```python
from build123d import *

# Parameters (mm, degrees)
SKETCH1_W                    = 129
SKETCH1_H                    = 107.4
SKETCH1_R                    = 1.65
BOSS_EXTRUDE1_DEPTH          = 3
BOSS_EXTRUDE2_DEPTH          = 5
BOSS_EXTRUDE3_START          = 5
SKETCH2_R                    = 4
SKETCH2_R_2                  = 1.6
BOSS_EXTRUDE3_DEPTH          = 5
CUT_EXTRUDE1_START           = 3
CUT_EXTRUDE1_OUTLINE_R       = 1.6
CUT_EXTRUDE1_DEPTH           = 2
FILLET3_R                    = 2
FILLET4_R                    = 2
SKETCH1_4_R                  = 2.407849471
CUT_EXTRUDE2_DEPTH           = 1
CUT_EXTRUDE2_DRAFT           = 45
CUT_EXTRUDE2_PROFILE_2_DEPTH = 1
CUT_EXTRUDE2_PROFILE_2_DRAFT = 45
CUT_EXTRUDE2_PROFILE_3_DEPTH = 1
CUT_EXTRUDE2_PROFILE_3_DRAFT = 45
CUT_EXTRUDE2_PROFILE_4_DEPTH = 1
CUT_EXTRUDE2_PROFILE_4_DRAFT = 45
CHAMFER1_SIZE                = 1.5


# Read off the part's stored shape, not the designer's step: Cut-Extrude1
with BuildPart() as part:
    # Sketch1 → Boss-Extrude1 (new body)
    with BuildSketch(Plane(origin=(0, 0, 0), x_dir=(1, 0, 0), z_dir=(0, 1, 0))):
        Rectangle(SKETCH1_W, SKETCH1_H)
        with Locations(Location((-60.3, -49.5, 0), (0, 0, 270))):
            Circle(SKETCH1_R, mode=Mode.SUBTRACT)
        with Locations(Location((60.3, -49.5, 0), (0, 0, 270))):
            Circle(SKETCH1_R, mode=Mode.SUBTRACT)
        with Locations(Location((-60.3, 49.5, 0), (0, 0, 270))):
            Circle(SKETCH1_R, mode=Mode.SUBTRACT)
        Polygon((49.912004588, -49.253731343), (-49.912004588, -49.253731343), (-60, -39.165735931), (-60, 39.165735931), (-49.912004588, 49.253731343), (49.912004588, 49.253731343), (60, 39.165735931), (60, -39.165735931), align=None, mode=Mode.SUBTRACT)
        with Locations(Location((60.3, 49.5, 0), (0, 0, 270))):
            Circle(SKETCH1_R, mode=Mode.SUBTRACT)
    extrude(amount=BOSS_EXTRUDE1_DEPTH)

    # Sketch1<3> → Boss-Extrude2 (add)
    with BuildSketch(Plane(origin=(0, 0, 0), x_dir=(1, 0, 0), z_dir=(0, 1, 0))):
        Polygon((-49.912004588, 49.253731343), (-60, 39.165735931), (-60, -39.165735931), (-49.912004588, -49.253731343), (49.912004588, -49.253731343), (60, -39.165735931), (60, 39.165735931), (49.912004588, 49.253731343), align=None)
    extrude(amount=BOSS_EXTRUDE2_DEPTH)

    # Sketch2 → Boss-Extrude3 (add)
    # profile 1 of 4: a face of its own
    with BuildSketch(Plane(origin=(0, 0, 0), x_dir=(1, 0, 0), z_dir=(0, 1, 0)).offset(BOSS_EXTRUDE3_START)):
        with Locations(Location((-39.313021369, -41.297235267, 0), (0, 0, 270))):
            Circle(SKETCH2_R)
        with Locations(Location((-39.313021369, -41.297235267, 0), (0, 0, 270))):
            Circle(SKETCH2_R_2, mode=Mode.SUBTRACT)
    # profile 2 of 4: a face of its own
    with BuildSketch(Plane(origin=(0, 0, 0), x_dir=(1, 0, 0), z_dir=(0, 1, 0)).offset(BOSS_EXTRUDE3_START)):
        with Locations(Location((36.886978631, 6.962764733, 0), (0, 0, 270))):
            Circle(SKETCH2_R)
        with Locations(Location((36.886978631, 6.962764733, 0), (0, 0, 270))):
            Circle(SKETCH2_R_2, mode=Mode.SUBTRACT)
    # profile 3 of 4: a face of its own
    with BuildSketch(Plane(origin=(0, 0, 0), x_dir=(1, 0, 0), z_dir=(0, 1, 0)).offset(BOSS_EXTRUDE3_START)):
        with Locations(Location((-38.043021369, 6.962764733, 0), (0, 0, 270))):
            Circle(SKETCH2_R)
        with Locations(Location((-38.043021369, 6.962764733, 0), (0, 0, 270))):
            Circle(SKETCH2_R_2, mode=Mode.SUBTRACT)
    # profile 4 of 4: a face of its own
    with BuildSketch(Plane(origin=(0, 0, 0), x_dir=(1, 0, 0), z_dir=(0, 1, 0)).offset(BOSS_EXTRUDE3_START)):
        with Locations(Location((43.236978631, -41.297235267, 0), (0, 0, 270))):
            Circle(SKETCH2_R)
        with Locations(Location((43.236978631, -41.297235267, 0), (0, 0, 270))):
            Circle(SKETCH2_R_2, mode=Mode.SUBTRACT)
    extrude(amount=BOSS_EXTRUDE3_DEPTH)

    # Cut-Extrude1 outline → Cut-Extrude1 (cut)
    with BuildSketch(Plane(origin=(0, 0, 0), x_dir=(1, 0, 0), z_dir=(0, 1, 0)).offset(CUT_EXTRUDE1_START)):
        with Locations((-38.043021369, 6.962764733)):
            Circle(CUT_EXTRUDE1_OUTLINE_R)
        with Locations((-39.313021369, -41.297235267)):
            Circle(CUT_EXTRUDE1_OUTLINE_R)
        with Locations((43.236978631, -41.297235267)):
            Circle(CUT_EXTRUDE1_OUTLINE_R)
        with Locations((36.886978631, 6.962764733)):
            Circle(CUT_EXTRUDE1_OUTLINE_R)
    extrude(amount=CUT_EXTRUDE1_DEPTH, mode=Mode.SUBTRACT)

    # Fillet3
    fillet3_edges = [part.edges().sort_by_distance(p)[0] for p in [
        (-54.956002294, 5, -44.209733637),
        (54.956002294, 5, -44.209733637),
        (0, 5, -49.253731343),
        (54.956002294, 5, 44.209733637),
        (60, 5, 0),
        (-60, 5, 0),
        (-54.956002294, 5, 44.209733637),
        (0, 5, 49.253731343),
    ]]
    fillet(fillet3_edges, radius=FILLET3_R - 0.0001)  # a hair under: the kernel refuses the full size

    # Fillet4
    fillet4_edges = [part.edges().sort_by_distance(p)[0] for p in [
        (-39.313021369, 5, 37.297235267),
        (43.236978631, 5, 37.297235267),
        (36.886978631, 5, -10.962764733),
        (-38.043021369, 5, -10.962764733),
    ]]
    fillet(fillet4_edges, radius=FILLET4_R)


with BuildPart() as cut_extrude2_tool:
    # Sketch1<4> → Cut-Extrude2 (with draft: the straight prism first)
    with BuildSketch(Plane(origin=(0, 0, 0), x_dir=(1, 0, 0), z_dir=(0, 1, 0))):
        with Locations((-60.3, 49.5)):
            Circle(SKETCH1_4_R)
    extrude(amount=CUT_EXTRUDE2_DEPTH)
    # Cut-Extrude2: the draft: its side faces are tilted about the plane it starts from
    cut_extrude2_sides = [cut_extrude2_tool.faces().sort_by_distance(p)[0] for p in [
        (-62.707849471, 0.5, -49.5),
    ]]
    draft(cut_extrude2_sides, Plane(origin=(0, 0, 0), x_dir=(1, 0, 0), z_dir=(0, 1, 0)), CUT_EXTRUDE2_DRAFT)


with BuildPart() as part_1:
    add(part.part)

    # Cut-Extrude2: cut by cut_extrude2_tool
    add(cut_extrude2_tool.part, mode=Mode.SUBTRACT)


with BuildPart() as cut_extrude2_profile_2_tool:
    # Sketch1<4> → Cut-Extrude2 profile 2 (with draft: the straight prism first)
    with BuildSketch(Plane(origin=(0, 0, 0), x_dir=(1, 0, 0), z_dir=(0, 1, 0))):
        with Locations((-60.3, -49.5)):
            Circle(SKETCH1_4_R)
    extrude(amount=CUT_EXTRUDE2_PROFILE_2_DEPTH)
    # Cut-Extrude2 profile 2: the draft: its side faces are tilted about the plane it starts from
    cut_extrude2_profile_2_sides = [cut_extrude2_profile_2_tool.faces().sort_by_distance(p)[0] for p in [
        (-62.707849471, 0.5, 49.5),
    ]]
    draft(cut_extrude2_profile_2_sides, Plane(origin=(0, 0, 0), x_dir=(1, 0, 0), z_dir=(0, 1, 0)), CUT_EXTRUDE2_PROFILE_2_DRAFT)


with BuildPart() as part_2:
    add(part_1.part)

    # Cut-Extrude2 profile 2: cut by cut_extrude2_profile_2_tool
    add(cut_extrude2_profile_2_tool.part, mode=Mode.SUBTRACT)


with BuildPart() as cut_extrude2_profile_3_tool:
    # Sketch1<4> → Cut-Extrude2 profile 3 (with draft: the straight prism first)
    with BuildSketch(Plane(origin=(0, 0, 0), x_dir=(1, 0, 0), z_dir=(0, 1, 0))):
        with Locations((60.3, -49.5)):
            Circle(SKETCH1_4_R)
    extrude(amount=CUT_EXTRUDE2_PROFILE_3_DEPTH)
    # Cut-Extrude2 profile 3: the draft: its side faces are tilted about the plane it starts from
    cut_extrude2_profile_3_sides = [cut_extrude2_profile_3_tool.faces().sort_by_distance(p)[0] for p in [
        (57.892150529, 0.5, 49.5),
    ]]
    draft(cut_extrude2_profile_3_sides, Plane(origin=(0, 0, 0), x_dir=(1, 0, 0), z_dir=(0, 1, 0)), CUT_EXTRUDE2_PROFILE_3_DRAFT)


with BuildPart() as part_3:
    add(part_2.part)

    # Cut-Extrude2 profile 3: cut by cut_extrude2_profile_3_tool
    add(cut_extrude2_profile_3_tool.part, mode=Mode.SUBTRACT)


with BuildPart() as cut_extrude2_profile_4_tool:
    # Sketch1<4> → Cut-Extrude2 profile 4 (with draft: the straight prism first)
    with BuildSketch(Plane(origin=(0, 0, 0), x_dir=(1, 0, 0), z_dir=(0, 1, 0))):
        with Locations((60.3, 49.5)):
            Circle(SKETCH1_4_R)
    extrude(amount=CUT_EXTRUDE2_PROFILE_4_DEPTH)
    # Cut-Extrude2 profile 4: the draft: its side faces are tilted about the plane it starts from
    cut_extrude2_profile_4_sides = [cut_extrude2_profile_4_tool.faces().sort_by_distance(p)[0] for p in [
        (57.892150529, 0.5, -49.5),
    ]]
    draft(cut_extrude2_profile_4_sides, Plane(origin=(0, 0, 0), x_dir=(1, 0, 0), z_dir=(0, 1, 0)), CUT_EXTRUDE2_PROFILE_4_DRAFT)


with BuildPart() as part_4:
    add(part_3.part)

    # Cut-Extrude2 profile 4: cut by cut_extrude2_profile_4_tool
    add(cut_extrude2_profile_4_tool.part, mode=Mode.SUBTRACT)

    # Chamfer1
    chamfer1_edges = [part_4.edges().sort_by_distance(p)[0] for p in [
        (0, 3, 53.7),
        (64.5, 3, 0),
        (0, 3, -53.7),
        (-64.5, 3, 0),
    ]]
    chamfer(chamfer1_edges, length=CHAMFER1_SIZE)


solid = part_4.part
```
Can you work these out from the model? Positions are in its coordinate system, mm. A direction names the side the tool comes from. Round coordinates to 2 decimals unless told otherwise and drop trailing zeros.
Item 1: Please list where these lines run through material, in increasing order: L1, parallel to Z at x = -60.3, y = 1.55; L2, parallel to Z at x = -60.3, y = 2.5; L3, parallel to Y at x = -53, z = 32.
Item 2: Which directions (+Z, -Z, +X, -X, +Y, -Y) give clear straight access to the entire face, cutting with the end or side of a thin tool? Please do faces 4 (the cylindrical face through (40.26, 8.48, -4.81)), 5 (the cylindrical face through (60.37, 1.86, -51.15)).
Item 3: If we mould it in two halves opening along X, with no side actions, what happens to faces 1 (the cylindrical face through (-36.63, 6.45, -6.21)), 2 (the flat face through (-40, 10, -7)), 3 (the cylindrical face through (-54.46, 4.43, 43.855))? For each: +X half, -X half, draft (parallel to the pull), parting line (faces both ways), or undercut.
Item 4: Will these pins go through, and if not, where does the flat tip stop? pin 1 Ø3 at (x, y) = (12, 5) entering from -Z; pin 2 Ø1 at (x, z) = (36, -7.5) entering from +Y; pin 3 Ø6 at (y, z) = (5.5, -28.5) entering from -X.
Reported:
1. L1: z = -53.65 to -51.15, -47.85 to 47.85, 51.15 to 53.65
1. L2: z = -52.7 to -51.15, -47.85 to 47.85, 51.15 to 52.7
1. L3: y = 0 to 5
2. face 4: +Y
2. face 5: +Y, -Y
3. face 1: undercut
3. face 2: draft
3. face 3: -X half
4. pin 1: stops at z = -49.19
4. pin 2: stops at y = 3
4. pin 3: stops at x = -63.5
